The model under review builds one solid part; all positions refer to its coordinate system, in mm. Face numbers are marked on the shaded views. A direction names the side the tool comes from. Give positions to 0.01 mm unless a question says otherwise; leave off trailing zeros. Order: outer loops, then holes, each group sorted by start corner. A loop starts at its lowest first (then second) coordinate and runs counter-clockwise, first axis right, second up. Notation, with made-up numbers: (67, 16.5) - (116, 16.5) arc R22 ccw to (116, 32.5) - close; hole circle Ø5 at (86, 75). An arc over 180 degrees is marked (long way). Write item = value, one per line. Start each with the question number.
1. We need section B-B, the plane z = 19. Give the boundary of the cut face in (x, y).
2. Wall thickness on probe 1 along Z at (x, y) = (-123.5, 75.25); probe 2 along Z at (x, y) = (-121.5, 66.75); probe 3 along X at (y, z) = (74.5, 15.5): over which ranges is each line inside the solid? List them lowest first.
3. Machinability: for the marked faces 4 and 5, which of the approach directions +Z, -Z, +X, -X, +Y, -Y give a long, thin tool a straight path to every point of the face, cutting with its end or side? Answer none if there is none.
4. We need section C-C, the plane x = -83. Give the boundary of the cut face in (y, z).
5. For P1, Ø5.5, axis at x = -84.5, z = 16.5, coming from the +Y side; P2, Ø10.5, axis at x = -84.82, z = -17.68, coming from the -Y side; P3, Ø3, axis at x = -63.5, y = 74, coming from the +Z side; P4, Ø4.5, axis at x = -63.39, y = 66, coming from the -Z side, all flat-tipped, find the tip position at first contact; note any pin that passes through.
6. We need section A-A, the plane y = 75. Give the boundary of the cut face in (x, z), and give its area (3 significant figures).
7. Mouldability with a two-part tool opening along Z and no side actions: class the marked faces 1, 2 and 3 as pulls with the +Z half, pulls with the -Z half, needs draft (parallel to the pull), parting line crosses it, or undercut.
8. We need section D-D, the plane y = 66. Give the boundary of the cut face in (x, z).
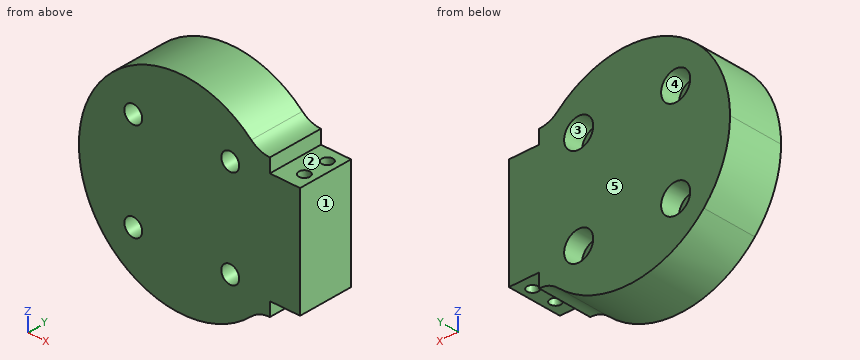
from build123d import *
from build123d.topology import SkipClean

# Parameters (mm, degrees)
SKETCH1_W                = 50
SKETCH1_H                = 50
SKETCH1_RX               = 19.7
SKETCH1_RY               = 19.1
BOSS_EXTRUDE1_DEPTH      = 35
SKETCH2_W                = 30
SKETCH2_H                = 50
CUT_EXTRUDE1_DEPTH       = 35
SKETCH3_W                = 13
SKETCH3_H                = 50
BOSS_EXTRUDE2_DEPTH      = 20
SKETCH4_R                = 1.5
CUT_EXTRUDE2_DEPTH       = 64.639610377
SKETCH5_W                = 36.974567712
SKETCH5_H                = 20
CUT_EXTRUDE3_DEPTH       = 20
BOSS_EXTRUDE3_DEPTH      = 4
BOSS_EXTRUDE3_DEPTH_BACK = 20
SKETCH6_W                = 14
SKETCH6_H                = 20
SKETCH6_R                = 3.25
SKETCH7_R                = 5.3
SKETCH7_R_2              = 3
CUT_EXTRUDE4_DEPTH       = 6
SKETCH8_W                = 13
SKETCH8_H                = 13.025432288
CUT_EXTRUDE5_DEPTH       = 30
FILLET6_R                = 4
FILLET5_R                = 10
SKETCH9_R                = 5.3
BOSS_EXTRUDE4_DEPTH      = 30
SKETCH10_W               = 20
SKETCH10_H               = 50
BOSS_EXTRUDE5_DEPTH      = 45
FILLET7_R                = 10
SKETCH11_W               = 50
SKETCH11_H               = 20
BOSS_EXTRUDE6_DEPTH      = 85
FILLET8_R                = 9.5
SKETCH13_R               = 37.5
BOSS_EXTRUDE7_DEPTH      = 20
CUT_EXTRUDE6_DEPTH       = 85
FILLET9_R                = 10
FILLET10_R               = 10
SKETCH14_R               = 3.25
CUT_EXTRUDE7_DEPTH       = 85
SKETCH15_R               = 5.3
CUT_EXTRUDE8_DEPTH       = 7
SKETCH16_R               = 3.25
BOSS_EXTRUDE9_DEPTH      = 36
SKETCH16_3_R             = 3.25
CUT_EXTRUDE11_DEPTH      = 10
SKETCH18_W               = 78
SKETCH18_H               = 80
CUT_EXTRUDE13_DEPTH      = 69.386919
SKETCH19_W               = 40
SKETCH19_H               = 20
BOSS_EXTRUDE10_DEPTH     = 11
SKETCH20_R               = 2
CUT_EXTRUDE14_DEPTH      = 9
CUT_EXTRUDE15_START      = -9
SKETCH21_R               = 2
CUT_EXTRUDE15_DEPTH      = 9


# Some blends are built 0.0001 mm under size
with BuildPart() as part:
    # Sketch1 → Boss-Extrude1 (new body)
    with BuildSketch(Plane(origin=(0, 0, 0), x_dir=(1, 0, 0), z_dir=(0, 1, 0))):
        Rectangle(SKETCH1_W, SKETCH1_H)
        with Locations((0, 0)):
            Ellipse(SKETCH1_RX, SKETCH1_RY, mode=Mode.SUBTRACT)
    extrude(amount=BOSS_EXTRUDE1_DEPTH)

    # Sketch2 → Cut-Extrude1 (cut)
    with BuildSketch(Plane(origin=(0, 35, 0), x_dir=(1, 0, 0), z_dir=(0, 1, 0))):
        with Locations((10, 0)):
            Rectangle(SKETCH2_W, SKETCH2_H)
    extrude(amount=-CUT_EXTRUDE1_DEPTH, mode=Mode.SUBTRACT)

    # Sketch3 → Boss-Extrude2 (add)
    with BuildSketch(Plane(origin=(0, 35, 0), x_dir=(1, 0, 0), z_dir=(0, 1, 0))):
        with Locations((-18.5, 0)):
            Rectangle(SKETCH3_W, SKETCH3_H)
    extrude(amount=BOSS_EXTRUDE2_DEPTH)

    # Sketch4 → Cut-Extrude2 (cut, through all)
    with BuildSketch(Plane.ZY.offset(25)):
        with Locations((18.474567712, 50)):
            Circle(SKETCH4_R)
    extrude(amount=-CUT_EXTRUDE2_DEPTH, mode=Mode.SUBTRACT)

    # Sketch5 → Cut-Extrude3 (cut)
    with BuildSketch(Plane(origin=(-12, 55, -25), x_dir=(0, 0, 1), z_dir=(-1, 0, 0))):
        with Locations((18.487283856, -10)):
            Rectangle(SKETCH5_W, SKETCH5_H)
    extrude(amount=CUT_EXTRUDE3_DEPTH, mode=Mode.SUBTRACT)

    # Sketch6 → Boss-Extrude3 (add, two sides: drawn at the far end of the back side and taken through both)
    # profile 1 of 2: a face of its own
    with BuildSketch(Plane(origin=(-5, 0, 0), x_dir=(0, 0, -1), z_dir=(1, 0, 0)).offset(-BOSS_EXTRUDE3_DEPTH_BACK)):
        with Locations((-32, 17.5)):
            Rectangle(SKETCH6_W, SKETCH6_H)
        with Locations((-32, 17.5)):
            Circle(SKETCH6_R, mode=Mode.SUBTRACT)
    # profile 2 of 2: a face of its own
    with BuildSketch(Plane(origin=(-5, 0, 0), x_dir=(0, 0, -1), z_dir=(1, 0, 0)).offset(-BOSS_EXTRUDE3_DEPTH_BACK)):
        with Locations((32, 17.5)):
            Rectangle(SKETCH6_W, SKETCH6_H)
        with Locations((32, 17.5)):
            Circle(SKETCH6_R, mode=Mode.SUBTRACT)
    extrude(amount=BOSS_EXTRUDE3_DEPTH + BOSS_EXTRUDE3_DEPTH_BACK)

    # Sketch7 → Cut-Extrude4 (cut)
    with BuildSketch(Plane.ZY.offset(25)):
        with Locations((-32, 17.5)):
            Circle(SKETCH7_R)
        with Locations((32, 17.5)):
            Circle(SKETCH7_R)
        with Locations((18.474567712, 50)):
            Circle(SKETCH7_R_2)
    extrude(amount=-CUT_EXTRUDE4_DEPTH, mode=Mode.SUBTRACT)

    # Sketch8 → Cut-Extrude5 (cut)
    with BuildSketch(Plane(origin=(0, 35, 0), x_dir=(1, 0, 0), z_dir=(0, 1, 0))):
        with Locations((-18.5, -18.487283856)):
            Rectangle(SKETCH8_W, SKETCH8_H)
    extrude(amount=CUT_EXTRUDE5_DEPTH, mode=Mode.SUBTRACT)

    # Fillet6
    fillet6_edges = [part.edges().sort_by_distance(p)[0] for p in [
        (-5, 17.5, 25),
        (-5, 17.5, -25),
    ]]
    fillet(fillet6_edges, radius=FILLET6_R - 0.0001)  # a hair under: the kernel refuses the full size

    # Fillet5
    # the kernel refuses this fillet: 10 mm, written as the material it adds along each edge
    with BuildSketch(Plane(origin=(-5, 7.5, 25), x_dir=(0, -1, 0), z_dir=(-1, 0, 0))) as fillet5_piece_1:
        with BuildLine():
            CenterArc((10, 9.682458366), FILLET5_R, 180, 75.522487814)
            Line((0, 9.682458366), (0, 0))
            Line((0, 0), (7.5, 0))
        make_face()
    extrude(amount=20)
    with BuildSketch(Plane(origin=(-5, 27.5, 25), x_dir=(0, 0, 1), z_dir=(-1, 0, 0)), Plane(origin=(-5, 7.5, -25), x_dir=(0, 0, -1), z_dir=(-1, 0, 0))) as fillet5_piece_2:
        with BuildLine():
            CenterArc((9.682458366, 10), FILLET5_R, 194.477512186, 75.522487814)
            Line((0, 7.5), (0, 0))
            Line((0, 0), (9.682458366, 0))
        make_face()
    extrude(amount=20)
    with BuildSketch(Plane(origin=(-5, 27.5, -25), x_dir=(0, 0, -1), z_dir=(-1, 0, 0))) as fillet5_piece_3:
        with BuildLine():
            CenterArc((9.682458366, -10), FILLET5_R, 90, 75.522487814)
            Line((0, -7.5), (0, 0))
            Line((0, 0), (9.682458366, 0))
        make_face()
    extrude(amount=20)

    # Sketch9 → Boss-Extrude4 (add)
    with BuildSketch(Plane.ZY.offset(25)):
        with BuildLine():
            Line((39, 27.5), (34.682458366, 27.5))
            ThreePointArc((34.682458366, 27.5), (28.558734009, 29.59430585), (25, 35))
            Line((25, 35), (-25, 35))
            ThreePointArc((-25, 35), (-28.558734009, 29.59430585), (-34.682458366, 27.5))
            Line((-34.682458366, 27.5), (-39, 27.5))
            Line((-39, 27.5), (-39, 7.5))
            Line((-39, 7.5), (-34.682458366, 7.5))
            ThreePointArc((-34.682458366, 7.5), (-28.558734009, 5.40569415), (-25, 0))
            Line((-25, 0), (25, 0))
            ThreePointArc((25, 0), (28.558734009, 5.40569415), (34.682458366, 7.5))
            Line((34.682458366, 7.5), (39, 7.5))
            Line((39, 7.5), (39, 27.5))
        make_face()
        with Locations((32, 17.5)):
            Circle(SKETCH9_R, mode=Mode.SUBTRACT)
        with Locations((-32, 17.5)):
            Circle(SKETCH9_R, mode=Mode.SUBTRACT)
    extrude(amount=BOSS_EXTRUDE4_DEPTH)

    # Sketch10 → Boss-Extrude5 (add)
    with SkipClean():  # the faces are left unmerged after this step: merging them gives an invalid solid
        with BuildSketch(Plane(origin=(0, 35, 0), x_dir=(1, 0, 0), z_dir=(0, 1, 0))):
            with Locations((-45, 0)):
                Rectangle(SKETCH10_W, SKETCH10_H)
        extrude(amount=BOSS_EXTRUDE5_DEPTH)

    # Fillet7
    fillet7_edges = [part.edges().sort_by_distance(p)[0] for p in [
        (-35, 35, 0),
    ]]
    fillet(fillet7_edges, radius=FILLET7_R - 0.0001)  # a hair under: the kernel refuses the full size

    # Sketch11 → Boss-Extrude6 (add)
    with BuildSketch(Plane.ZY.offset(55)):
        with Locations((0, 70)):
            Rectangle(SKETCH11_W, SKETCH11_H)
    extrude(amount=BOSS_EXTRUDE6_DEPTH)

    # Fillet8
    fillet8_edges = [part.edges().sort_by_distance(p)[0] for p in [
        (-55, 60, 0),
    ]]
    fillet(fillet8_edges, radius=FILLET8_R)

    # Sketch13 → Boss-Extrude7 (add)
    with BuildSketch(Plane(origin=(0, 80, 0), x_dir=(1, 0, 0), z_dir=(0, 1, 0))):
        with Locations((-102.5, 0)):
            Circle(SKETCH13_R)
    extrude(amount=-BOSS_EXTRUDE7_DEPTH)

    # Sketch13<3> → Cut-Extrude6 (cut)
    with BuildSketch(Plane(origin=(0, 80, 0), x_dir=(1, 0, 0), z_dir=(0, 1, 0))):
        with BuildLine():
            Line((-124.371968295, 30.460909424), (-140, 25))
            Line((-140, 25), (-140, 0))
            ThreePointArc((-140, 0), (-135.865017691, 17.117990375), (-124.371968295, 30.460909424))
        make_face()
        with BuildLine():
            ThreePointArc((-130.450849719, -25), (-137.531463461, -13.380828366), (-140, 0))
            Line((-140, 0), (-140, -25))
            Line((-140, -25), (-130.450849719, -25))
        make_face()
    extrude(amount=-CUT_EXTRUDE6_DEPTH, mode=Mode.SUBTRACT)

    # Fillet9
    fillet9_edges = [part.edges().sort_by_distance(p)[0] for p in [
        (-74.549150281, 70, 25),
        (-74.549150281, 70, -25),
    ]]
    fillet(fillet9_edges, radius=FILLET9_R)

    # Fillet10
    fillet10_edges = [part.edges().sort_by_distance(p)[0] for p in [
        (-35, 80, 0),
    ]]
    fillet(fillet10_edges, radius=FILLET10_R)

    # Sketch14 → Cut-Extrude7 (cut)
    with BuildSketch(Plane(origin=(0, 80, 0), x_dir=(1, 0, 0), z_dir=(0, 1, 0))):
        with Locations(Location((-120.17766953, 17.67766953, 0), (0, 0, 270))):
            Circle(SKETCH14_R)
        with Locations(Location((-120.17766953, -17.67766953, 0), (0, 0, 270))):
            Circle(SKETCH14_R)
        with Locations(Location((-84.82233047, -17.67766953, 0), (0, 0, 270))):
            Circle(SKETCH14_R)
        with Locations(Location((-84.82233047, 17.67766953, 0), (0, 0, 270))):
            Circle(SKETCH14_R)
    extrude(amount=-CUT_EXTRUDE7_DEPTH, mode=Mode.SUBTRACT)

    # Sketch15 → Cut-Extrude8 (cut)
    with BuildSketch(Plane(origin=(0, 80, 0), x_dir=(1, 0, 0), z_dir=(0, 1, 0))):
        with Locations(Location((-120.17766953, 17.67766953, 0), (0, 0, 270))):
            Circle(SKETCH15_R)
        with Locations(Location((-120.17766953, -17.67766953, 0), (0, 0, 270))):
            Circle(SKETCH15_R)
        with Locations(Location((-84.82233047, -17.67766953, 0), (0, 0, 270))):
            Circle(SKETCH15_R)
        with Locations(Location((-84.82233047, 17.67766953, 0), (0, 0, 270))):
            Circle(SKETCH15_R)
    extrude(amount=-CUT_EXTRUDE8_DEPTH, mode=Mode.SUBTRACT)

    # Sketch16 → Boss-Extrude9 (add)
    # profile 1 of 2: a face of its own
    with BuildSketch(Plane.ZY.offset(55)):
        Polygon((-25.937822174, 17.5), (-28.968911087, 22.75), (-35.031088913, 22.75), (-38.062177826, 17.5), (-35.031088913, 12.25), (-28.968911087, 12.25), align=None)
        with Locations(Location((-32, 17.5, 0), (0, 0, 180))):
            Circle(SKETCH16_R, mode=Mode.SUBTRACT)
    # profile 2 of 2: a face of its own
    with BuildSketch(Plane.ZY.offset(55)):
        Polygon((25.937822174, 17.5), (28.968911087, 12.25), (35.031088913, 12.25), (38.062177826, 17.5), (35.031088913, 22.75), (28.968911087, 22.75), align=None)
        with Locations(Location((32, 17.5, 0), (0, 0, 180))):
            Circle(SKETCH16_R, mode=Mode.SUBTRACT)
    extrude(amount=-BOSS_EXTRUDE9_DEPTH)

    # Sketch16<3> → Cut-Extrude11 (cut)
    # profile 1 of 2: a face of its own
    with BuildSketch(Plane.ZY.offset(55)):
        Polygon((-25.937822174, 17.5), (-28.968911087, 22.75), (-35.031088913, 22.75), (-38.062177826, 17.5), (-35.031088913, 12.25), (-28.968911087, 12.25), align=None)
        with Locations(Location((-32, 17.5, 0), (0, 0, 180))):
            Circle(SKETCH16_3_R, mode=Mode.SUBTRACT)
    # profile 2 of 2: a face of its own
    with BuildSketch(Plane.ZY.offset(55)):
        Polygon((25.937822174, 17.5), (28.968911087, 12.25), (35.031088913, 12.25), (38.062177826, 17.5), (35.031088913, 22.75), (28.968911087, 22.75), align=None)
        with Locations(Location((32, 17.5, 0), (0, 0, 180))):
            Circle(SKETCH16_3_R, mode=Mode.SUBTRACT)
    extrude(amount=-CUT_EXTRUDE11_DEPTH, mode=Mode.SUBTRACT)

    # Sketch18 → Cut-Extrude13 (cut)
    with BuildSketch(Plane(origin=(-1, 0, 0), x_dir=(0, 0, -1), z_dir=(1, 0, 0))):
        with Locations((0, 40)):
            Rectangle(SKETCH18_W, SKETCH18_H)
    extrude(amount=-CUT_EXTRUDE13_DEPTH, mode=Mode.SUBTRACT)


with BuildPart() as boss_extrude10_tool:
    # Sketch19 → Boss-Extrude10 (new body)
    with BuildSketch(Plane(origin=(-70.386918553, 0, 0), x_dir=(0, 0, -1), z_dir=(1, 0, 0))):
        with Locations((0, 70)):
            Rectangle(SKETCH19_W, SKETCH19_H)
    extrude(amount=BOSS_EXTRUDE10_DEPTH)


with BuildPart() as part_1:
    add(part.part)


with BuildPart() as part_2:
    # Boss-Extrude10: joined with boss_extrude10_tool
    add(part_1.part.fuse(boss_extrude10_tool.part, tol=0.00001))

    # Sketch20 → Cut-Extrude14 (cut)
    with BuildSketch(Plane.XY.offset(20)):
        with Locations((-63.386918553, 75)):
            Circle(SKETCH20_R)
        with Locations((-63.386918553, 66)):
            Circle(SKETCH20_R)
    extrude(amount=-CUT_EXTRUDE14_DEPTH, mode=Mode.SUBTRACT)

    # Sketch21 → Cut-Extrude15 (cut)
    with BuildSketch(Plane(origin=(0, 0, -20), x_dir=(-1, 0, 0), z_dir=(0, 0, -1)).offset(CUT_EXTRUDE15_START)):
        with Locations(Location((63.386918553, 75, 0), (0, 0, 180))):
            Circle(SKETCH21_R)
        with Locations(Location((63.386918553, 66, 0), (0, 0, 180))):
            Circle(SKETCH21_R)
    extrude(amount=CUT_EXTRUDE15_DEPTH, mode=Mode.SUBTRACT)


solid = part_2.part
Model answer:
q1.outline = (-134.83, 60) - (-123.15, 60) - (-123.15, 73) - (-125.31, 73) - (-125.31, 80) - (-134.83, 80) - close; (-117.21, 60) - (-87.79, 60) - (-87.79, 73) - (-89.95, 73) - (-89.95, 80) - (-115.05, 80) - (-115.05, 73) - (-117.21, 73) - close; (-81.85, 60) - (-59.39, 60) - (-59.39, 80) - (-79.69, 80) - (-79.69, 73) - (-81.85, 73) - close; hole circle Ø4 at (-63.39, 66); hole circle Ø4 at (-63.39, 75)
q2.probe_1 = -31.07 to -21.81, -13.55 to 13.55, 21.81 to 31.07
q2.probe_2 = -32.33 to -20.65, -14.71 to 14.71, 20.65 to 32.33
q2.probe_3 = -136.65 to -125.01, -115.35 to -89.65, -79.99 to -65.32, -61.45 to -59.39
q3.face_4 = +Y
q3.face_5 = +Z, -Z, +X, -X, +Y
q4.outline = (60, -32.03) - (80, -32.03) - (80, -22.65) - (73, -22.65) - (73, -20.37) - (60, -20.37) - close; (60, -14.99) - (73, -14.99) - (73, -12.7) - (80, -12.7) - (80, 12.7) - (73, 12.7) - (73, 14.99) - (60, 14.99) - close; (60, 20.37) - (73, 20.37) - (73, 22.65) - (80, 22.65) - (80, 32.03) - (60, 32.03) - close
q5.P1 = 73
q5.P2 = 60
q5.P3 = 20
q5.P4 = -20
q6.outline = (-77.15, -27.63) arc R10 cw to (-70.39, -25) - (-70.39, -20) - (-65.39, -20) - (-65.39, -11) - (-61.39, -11) - (-61.39, -20) - (-59.39, -20) - (-59.39, 20) - (-61.39, 20) - (-61.39, 11) - (-65.39, 11) - (-65.39, 20) - (-70.39, 20) - (-70.39, 25) arc R10 cw to (-77.15, 27.63) arc R37.5 ccw (long way) to start; hole circle Ø10.6 at (-120.18, -17.68); hole circle Ø10.6 at (-120.18, 17.68); hole circle Ø10.6 at (-84.82, -17.68); hole circle Ø10.6 at (-84.82, 17.68)
q6.area = 4,320 mm2
q7.face_1 = needs draft
q7.face_2 = pulls with the +Z half
q7.face_3 = undercut
q8.outline = (-77.15, -27.63) arc R10 cw to (-70.39, -25) - (-70.39, -20) - (-65.39, -20) - (-65.39, -11) - (-61.39, -11) - (-61.39, -20) - (-59.39, -20) - (-59.39, 20) - (-61.39, 20) - (-61.39, 11) - (-65.39, 11) - (-65.39, 20) - (-70.39, 20) - (-70.39, 25) arc R10 cw to (-77.15, 27.63) arc R37.5 ccw (long way) to start; hole circle Ø6.5 at (-120.18, -17.68); hole circle Ø6.5 at (-120.18, 17.68); hole circle Ø6.5 at (-84.82, -17.68); hole circle Ø6.5 at (-84.82, 17.68)
